```python
from build123d import *

# Parameters (mm, degrees)
CROQUIS1_W              = 1.4
CROQUIS1_H              = 4.5
SALIENTE_EXTRUIR1_DEPTH = 4.65
CROQUIS2_W              = 0.51
CROQUIS2_H              = 0.51
SALIENTE_EXTRUIR2_DEPTH = 12.7


with BuildPart() as part:
    # Croquis1 → Saliente-Extruir1 (new body)
    with BuildSketch(Plane(origin=(0, 0, 0), x_dir=(1, 0, 0), z_dir=(0, 1, 0))):
        with Locations((0.7, 2.25)):
            Rectangle(CROQUIS1_W, CROQUIS1_H)
    extrude(amount=SALIENTE_EXTRUIR1_DEPTH)

    # Croquis2 → Saliente-Extruir2 (add)
    with BuildSketch(Plane.XZ):
        with Locations((0.7, -1)):
            Rectangle(CROQUIS2_W, CROQUIS2_H)
        with Locations((0.7, -3.5)):
            Rectangle(CROQUIS2_W, CROQUIS2_H)
    extrude(amount=SALIENTE_EXTRUIR2_DEPTH)


solid = part.part
```
Input: part model. Units: mm. Frame: model coordinates. Round coordinates to 2 decimals unless told otherwise and drop trailing zeros. Loops run counter-clockwise (first coordinate to the right, second up) from the corner with the lowest first, then second, coordinate; pieces in that order, holes last. Notation, with made-up numbers: (1, 26.25) -> (45, 26.25) arc R16 ccw to (45, 43.25) -> close; hole circle Ø6 at (40.5, 44.5). An arc over 180 degrees is marked (long way). Use one line per item in the form item = value. Start each with the question number.
Item 1: Contact query for flat-ended pins moving along their axis: pin 1 Ø0.6 at (x, y) = (0.5, -4.5) entering from -Z (3 decimals); pin 2 Ø2 at (y, z) = (-7, -1) entering from +X (3 decimals). Output: stop coordinate, or through.
Item 2: Section query B-B on x = 0.6. Return the cut outline in (y, z) (3 decimals).
Item 3: Section query A-A on y = -3.5. Return the cut outline in (x, z) (3 decimals), then the cut area to 3 significant figures.
Item 4: Section query C-C on z = -1.6. Return the cut outline in (x, y).
Item 5: Material intervals for L1, parallel to Z at x = 0.6, y = -3.25 (3 decimals); L2, parallel to Y at x = 0.7, z = -1.3; L3, parallel to X at y = -8.25, z = -1 (3 decimals), sorted ascending. Write a range as from..to.
Item 6: Mould query, pull axis Z, two halves, no side actions, for faces 1 (the face through (1, 4.65, -2)), 2 (the face through (1, 2, -4.5)), 3 (the face through (1, 0, -2)). Classes: pulls with the +Z half, pulls with the -Z half, needs draft (parallel to the pull), parting line crosses it, or undercut.
Ans:
q1.pin_1 = -3.755
q1.pin_2 = 0.955
q2.outline = (-12.7, -3.755) -> (0, -3.755) -> (0, -4.5) -> (4.65, -4.5) -> (4.65, 0) -> (0, 0) -> (0, -0.745) -> (-12.7, -0.745) -> (-12.7, -1.255) -> (0, -1.255) -> (0, -3.245) -> (-12.7, -3.245) -> close
q3.outline = (0.445, -3.755) -> (0.955, -3.755) -> (0.955, -3.245) -> (0.445, -3.245) -> close; (0.445, -1.255) -> (0.955, -1.255) -> (0.955, -0.745) -> (0.445, -0.745) -> close
q3.area = 0.520 mm^2
q4.outline = (0, 0) -> (1.4, 0) -> (1.4, 4.65) -> (0, 4.65) -> close
q5.L1 = -3.755..-3.245, -1.255..-0.745
q5.L2 = 0..4.65
q5.L3 = 0.445..0.955
q6.face_1 = needs draft
q6.face_2 = pulls with the -Z half
q6.face_3 = undercut
